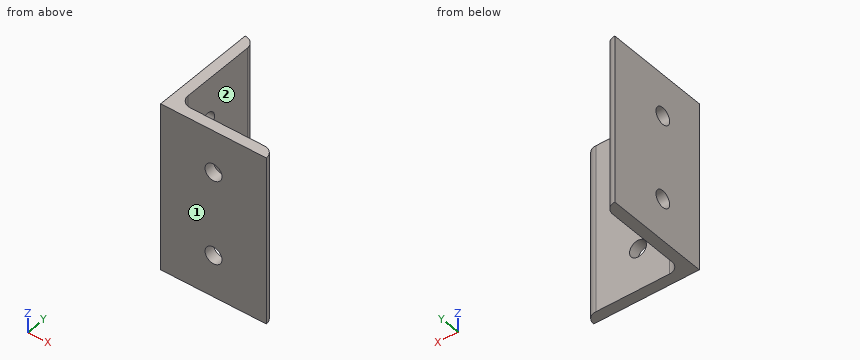
from build123d import *

# Parameters (mm, degrees)
BOSS_EXTRUDE1_DEPTH = 25.4
SKETCH2_R           = 2.5527
CUT_EXTRUDE1_DEPTH  = 52.587643869
SKETCH3_R           = 2.5527
CUT_EXTRUDE2_DEPTH  = 52.587643869
FILLET1_R           = 3.175


with BuildPart() as part:
    # Sketch1 → Boss-Extrude1 (new, symmetric)
    with BuildSketch(Plane.XY):
        Polygon((0, 0), (0, 31.75), (3.175, 31.75), (3.175, 3.175), (31.75, 3.175), (31.75, 0), align=None)
    extrude(amount=BOSS_EXTRUDE1_DEPTH, both=True)

    # Sketch2 → Cut-Extrude1 (cut, through all)
    with BuildSketch(Plane.ZY):
        with Locations((-12.7, 13.716)):
            Circle(SKETCH2_R)
        with Locations((12.7, 13.716)):
            Circle(SKETCH2_R)
    extrude(amount=-CUT_EXTRUDE1_DEPTH, mode=Mode.SUBTRACT)

    # Sketch3 → Cut-Extrude2 (cut, through all)
    with BuildSketch(Plane.XZ):
        with Locations(Location((15.875, 12.7, 0), (0, 0, 270))):
            Circle(SKETCH3_R)
        with Locations(Location((15.875, -12.7, 0), (0, 0, 270))):
            Circle(SKETCH3_R)
    extrude(amount=-CUT_EXTRUDE2_DEPTH, mode=Mode.SUBTRACT)

    # Fillet1
    fillet1_edges = [part.edges().sort_by_distance(p)[0] for p in [
        (3.175, 31.75, 0),
        (31.75, 3.175, 0),
        (3.175, 3.175, 0),
    ]]
    fillet(fillet1_edges, radius=FILLET1_R - 0.0001)  # a hair under: the kernel refuses the full size


solid = part.part
Here's how the part is built. I have some questions about the finished solid (model axes, mm). Face numbers are marked on the shaded views. A direction names the side the tool comes from. Coordinates: 2 decimals unless noted, no trailing zeros. Order: outer loops, then holes, each group sorted by start corner. A loop starts at its lowest first (then second) coordinate and runs counter-clockwise, first axis right, second up.
Item 1: I need wall thicknesses on line 1 (Y direction, x = 7, z = -13) (3 decimals); line 2 (X direction, y = 1, z = -12.7). Which ranges of each line are inside material? Lowest first, please.
Result sheet:
line 1: y = 0 to 3.175
line 2: x = 0 to 13.32, 18.43 to 31.59
Item 2: If we section it at C-C on x = 17: List the corners of the cut face in (y, z) for me (3 decimals), plus the area to 3 significant figures.
Result sheet:
outline: (0, -25.4) - (3.175, -25.4) - (3.175, -14.991) - (0, -14.991) - close; (0, -10.409) - (3.175, -10.409) - (3.175, 10.409) - (0, 10.409) - close; (0, 14.991) - (3.175, 14.991) - (3.175, 25.4) - (0, 25.4) - close
area: 132 mm2
Item 3: For P1, Ø6.5, axis at x = 18, z = 1, coming from the +Y side (3 decimals); P2, Ø6, axis at y = 25, z = 2, coming from the -X side; P3, Ø18, axis at y = 13, z = -11, coming from the +X side; P4, Ø5, axis at x = 3.5, z = 19, coming from the +Y side, each with a flat end and sliding along its axis, tell me the tip position at first contact or that it passes through.
Result sheet:
P1: stops at y = 3.175
P2: stops at x = 0
P3: stops at x = 4.21
P4: stops at y = 31.59
Item 4: If we section it at D-D on y = 2: List the corners of the cut face in (x, z) for me (3 decimals).
Result sheet:
outline: (0, -25.4) - (31.041, -25.4) - (31.041, 25.4) - (0, 25.4) - close; hole circle Ø5.105 at (15.875, -12.7); hole circle Ø5.105 at (15.875, 12.7)
Item 5: For the marked faces 1 and 2, which set-ups out of +Z, -Z, +X, -X, +Y, -Y let a thin tool reach every point of the face, with its end or its side?
Result sheet:
face 1: +Z, -Z, +X, -X, -Y
face 2: +Z, -Z, +X, +Y
Item 6: If we section it at A-A on z = 12.7: State how many separate pieces and enclosed holes the cut face has, plus the area to 3 significant figures.
Result sheet:
separate pieces: 3
enclosed holes: 0
area: 157 mm2
